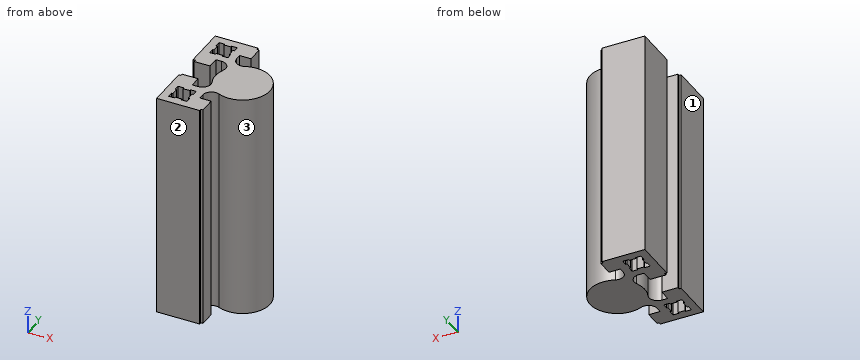
Autodesk Inventor part; units mm, degrees
ref_plane "YZ Plane" through (0, 0, 0) normal (1, 0, 0) x (0, 1, 0)
ref_plane "XZ Plane" through (0, 0, 0) normal (0, 1, 0) x (-1, 0, 0)
ref_plane "XY Plane" through (0, 0, 0) normal (0, 0, 1) x (1, 0, 0)
sketch "Sketch1" plane through (0, 0, 0) normal (0, 0, 1) x (1, 0, 0)
  circle A0 centre (-25, 0) radius 6
  line L0 (0, 0) -> (-25, 0) construction
  circle A1 centre (-25, 0) radius 12
  line L1 (-45.9, 14.1) -> (-39.1, 14.1) construction
  line L2 (-39.1, 14.1) -> (-39.1, 20.9) construction
  line L3 (-39.1, 20.9) -> (-45.9, 20.9) construction
  line L4 (-45.9, 20.9) -> (-45.9, 14.1) construction
  line L5 (-45.9, 14.1) -> (-39.1, 20.9) construction
  line L6 (-39.1, 14.1) -> (-45.9, 20.9) construction
  line L7 (-46.5, 13.5) -> (-38.5, 13.5) construction
  line L8 (-38.5, 13.5) -> (-38.5, 21.5) construction
  line L9 (-38.5, 21.5) -> (-46.5, 21.5) construction
  line L10 (-46.5, 21.5) -> (-46.5, 13.5) construction
  line L11 (-46.5, 13.5) -> (-38.5, 21.5) construction
  line L12 (-38.5, 13.5) -> (-46.5, 21.5) construction
  line L13 (-44, 20.9) -> (-41, 20.9)
  line L14 (-44, 20.9) -> (-44, 21.5)
  line L15 (-44, 21.5) -> (-46.5, 21.5)
  line L16 (-41, 20.9) -> (-41, 21.5)
  line L17 (-41, 21.5) -> (-38.5, 21.5)
  line L18 (-46.5, 21.5) -> (-46.5, 19)
  line L19 (-46.5, 19) -> (-45.9, 19)
  line L20 (-45.9, 19) -> (-45.9, 16)
  line L21 (-45.9, 16) -> (-46.5, 16)
  line L22 (-46.5, 16) -> (-46.5, 13.5)
  line L23 (-46.5, 13.5) -> (-44, 13.5)
  line L24 (-44, 13.5) -> (-44, 14.1)
  line L25 (-44, 14.1) -> (-41, 14.1)
  line L26 (-41, 14.1) -> (-41, 13.5)
  line L27 (-41, 13.5) -> (-38.5, 13.5)
  line L28 (-38.5, 13.5) -> (-38.5, 16)
  line L29 (-38.5, 16) -> (-39.1, 16)
  line L30 (-39.1, 16) -> (-39.1, 19)
  line L31 (-39.1, 19) -> (-38.5, 19)
  line L32 (-38.5, 19) -> (-38.5, 21.5)
  line L33 (-50, 25) -> (-50, 5.1) construction
  line L34 (-50, 25) -> (-30.1, 25) construction
  line L35 (-50, 5.1) -> (-49, 5.1) construction
  line L36 (-49, 5.1) -> (-49, 6.1)
  line L37 (-49, 6.1) -> (-50, 6.1)
  line L38 (-50, 6.1) -> (-50, 5.1) construction
  line L39 (-50, 5.1) -> (-49, 6.1) construction
  line L40 (-49, 5.1) -> (-50, 6.1) construction
  line L41 (-50, 6.1) -> (-50, 25)
  line L42 (-31.1, 24) -> (-30.1, 24)
  line L43 (-30.1, 24) -> (-30.1, 25) construction
  line L44 (-30.1, 25) -> (-31.1, 25) construction
  line L45 (-31.1, 25) -> (-31.1, 24)
  line L46 (-31.1, 24) -> (-30.1, 25) construction
  line L47 (-30.1, 24) -> (-31.1, 25) construction
  line L48 (-50, 25) -> (-31.1, 25)
  line L49 (-30.1, 24) -> (-30.1, 17)
  line L50 (-30.1, 17) -> (-35.1, 17)
  line L51 (-35.1, 17) -> (-35.1, 12) construction
  line L52 (-35.1, 12) -> (-25, 12) construction
  arc A2 (-35.1, 14.5) -> (-29.7776, 11.0079) centre (-31.2932, 14.5) ccw
  line L53 (-35.1, 17) -> (-35.1, 14.5)
  line L54 (-49, 5.1) -> (-42, 5.1)
  line L55 (-42, 5.1) -> (-42, 10.1)
  line L56 (-42, 10.1) -> (-39.5, 10.1)
  arc A3 (-36.0079, 4.7776) -> (-39.5, 10.1) centre (-39.5, 6.2932) ccw
  arc A4 (-20.2224, 11.0079) -> (-14.9, 14.5) centre (-18.7068, 14.5) ccw
  line L57 (-14.9, 14.5) -> (-14.9, 17)
  line L58 (-14.9, 17) -> (-19.9, 17)
  line L59 (-19.9, 17) -> (-19.9, 24)
  line L60 (-19.9, 24) -> (-18.9, 24)
  line L61 (-18.9, 24) -> (-18.9, 25)
  line L62 (-18.9, 25) -> (-19.9, 25) construction
  line L63 (-19.9, 25) -> (-19.9, 24) construction
  line L64 (-19.9, 24) -> (-18.9, 25) construction
  line L65 (-18.9, 24) -> (-19.9, 25) construction
  line L66 (-18.9, 25) -> (0, 25)
  line L67 (0, 22) -> (-11.9, 22) construction
  line L68 (-11.9, 22) -> (-11.9, 14.5) construction
  line L69 (0, 22) -> (0, 25)
  arc A5 (-10.9, 22) -> (-11.9, 21) centre (-10.9, 21) ccw
  line L70 (-11.9, 21) -> (-11.9, 14.5)
  line L71 (-10.9, 22) -> (0, 22)
  arc A6 (-13.1902, 10.8149) -> (-13.9921, 4.7776) centre (-8.5727, 7.1297) ccw
  arc A7 (-13.1902, 10.8149) -> (-11.9, 14.5) centre (-17.8078, 14.5) ccw
  point P0 (-42.5, 17.5)
  point P1 (-42.5, 17.5)
  point P2 (-42.5, 17.5)
  point P3 (-42.5, 20.9)
  point P4 (-49.5, 5.6)
  point P5 (-30.6, 24.5)
  point P6 (-19.4, 24.5)
  dimension "d0" = 25
  dimension "d1" = 12
  dimension "d2" = 24
  dimension "d16" = 17.5
  dimension "d17" = 42.5
  dimension "d18" = 6.8
  dimension "d19" = 8
  dimension "d20" = 3
  dimension "d21" = 5.1
  dimension "d22" = 25
  dimension "d23" = 50
  dimension "d24" = 1
  dimension "d25" = 7
  dimension "d26" = 5
  dimension "d27" = 5
  dimension "d30" = 3
  dimension "d31" = 3
  dimension "d34" = 1
extrude "Extrusion1" add sketch "Sketch1" along normal mid plane 100 contours A1
sketch "Sketch2" plane through (-25, 0, 50) normal (0, 0, 1) x (1, 0, 0)
  circle A0 centre (0, 0) radius 6 construction
  line L0 (0, 0) -> (1.3656, 6.8655) construction
  circle A1 centre (0, 0) radius 7 construction
  line L1 (0, 0) -> (-1.3656, 6.8655) construction
  line L2 (0, 0) -> (0, 7) construction
  line L3 (0, 0) -> (-3.889, 5.8203) construction
  arc A2 (-1.1705, 5.8847) -> (-3.3334, 4.9888) centre (0, 0) ccw
  line L4 (-3.3334, 4.9888) -> (-3.889, 5.8203)
  line L5 (-1.1705, 5.8847) -> (-1.3656, 6.8655)
  arc A3 (-1.3656, 6.8655) -> (-3.889, 5.8203) centre (0, 0) ccw
  point P0 (25, 0)
  point P1 (-2.6788, 6.4672)
  dimension "d5" = 14
  dimension "d6" = 22.5
  dimension "d7" = 22.5
extrude "Extrusion2" cut sketch "Sketch2" against normal through all
pattern_circular "Circular Pattern2" count 8 over 360 about axis through (-25, 0, 0) along (0, 0, 1) of "Extrusion2"
extrude "Extrusion3" add sketch "Sketch1" along normal mid plane 100 contours A3 L56 L55 L54 L36 L37 L41 L48 L45 L42 L49 L50 L53 A2 A1
mirror "Mirror1" about plane through (0, 0, 0) normal (0, 1, 0) of "Extrusion3"
extrude "Extrusion4" add sketch "Sketch1" along normal mid plane 100 contours A0 | A1
equation "\"d31\" = d30"
equation "\"d7\" = d6"
properties part number "perfil-aluminio-0002-001"
For this review, take the finished solid that the model builds, in its own axes (mm). Face numbers are marked on the shaded views. Round coordinates to 2 decimals unless told otherwise and drop trailing zeros. Loops run counter-clockwise (first coordinate to the right, second up) from the corner with the lowest first, then second, coordinate; pieces in that order, holes last. Notation, with made-up numbers: (27.25, -7.5) - (76.25, -7.5) arc R23 cw to (76.25, 25.5) - close; hole circle Ø4 at (33.25, -33). An arc over 180 degrees is marked (long way). Use one line per item in the form item = value.
Item 1: Consider section A-A on y = 0. Write out the cut boundary in (x, z), then the cut area to 3 significant figures.
Answers:
outline = (-37, -50) - (-13, -50) - (-13, 50) - (-37, 50) - close
area = 2,400 mm^2
Item 2: Consider section C-C on z = 21.5. State how many separate pieces and enclosed holes the cut face has, then the cut area to 3 significant figures.
Answers:
separate_pieces = 1
enclosed_holes = 2
area = 972 mm^2
Item 3: For line 1 (X direction, y = 20, z = -2); line 2 (X direction, y = -17.5, z = -30.5); line 3 (Y direction, x = -43, z = -28), list the stretches that pass through material, from the lowest coordinate up.
Answers:
line_1 = -50 to -46.5, -38.5 to -30.1
line_2 = -50 to -45.9, -39.1 to -30.1
line_3 = -25 to -20.9, -14.1 to -5.1, 5.1 to 14.1, 20.9 to 25
Item 4: Clearance check with flat-ended pins moving along their axes: P1, Ø5, axis at x = -25.5, z = 2, coming from the -Y side; P2, Ø0.5, axis at y = -21, z = -2.5, coming from the +X side; P3, Ø8, axis at y = -3.5, z = -30.5, coming from the -X side; P4, Ø2, axis at y = -14.5, z = 4, coming from the +X side. State where each tip first meets the part, or that it passes through.
Answers:
P1 = -12
P2 = -30.1
P3 = -50
P4 = -34.97
Item 5: Mouldability with a two-part tool opening along X and no side actions: class the marked faces 1, 2 and 3 as +X half, -X half, draft (parallel to the pull), parting line (faces both ways), or undercut.
Answers:
face_1 = -X half
face_2 = draft
face_3 = undercut
Item 6: Consider section B-B on x = -25. Write out the cut boundary in (y, z), then the cut area to 3 significant figures.
Answers:
outline = (-12, -50) - (12, -50) - (12, 50) - (-12, 50) - close
area = 2,400 mm^2
